Can you work these out from the model? Positions are in its coordinate system, mm. A direction names the side the tool comes from. Give positions to 0.01 mm unless a question says otherwise; leave off trailing zeros. Order: outer loops, then holes, each group sorted by start corner. A loop starts at its lowest first (then second) coordinate and runs counter-clockwise, first axis right, second up. Notation, with made-up numbers: M 75.5,81 L 119.5,81 A16 ccw 119.5,101 Z; hole C -9.5,-17 d2. An arc over 180 degrees is marked long. One line per question, with ' | ' between items. Start each with the question number.
1) If we section it at A-A, the plane y = 67.5: Please give me the cut outline in (x, z).
2) If we section it at D-D, the plane y = 79: Please give me the cut outline in (x, z), plus the area to 3 significant figures.
3) If we section it at C-C, the plane x = -25: State how many separate pieces and enclosed holes the cut face has, plus the area to 3 significant figures.
4) Thinking about a two-plate mould opening in Z: for faces 5 (the flat face through (-57.2, 19, 178)), 6 (the flat face through (-55.93, 24.31, 181.27)), which applies, +Z half, -Z half, draft (parallel to the pull), parting line (faces both ways), or undercut?
5) If we section it at B-B, the plane z = 65.5: Please give me the cut outline in (x, y).
6) For faces 1 (the flat face through (-55.932, 18.14, 98.395)), 2 (the flat face through (-1, 27, 169)), 3 (the flat face through (56.132, 24.308, 242.731)), 4 (the conical face through (-36.364, 61.607, -2.188)), which set-ups out of +Z, -Z, +X, -X, +Y, -Y let a thin tool reach every point of the face, with its end or its side?
7) I'm going to push flat-ended pins straight in: pin 1 Ø3 at (x, z) = (38.5, 98.5) entering from +Y; pin 2 Ø2.5 at (y, z) = (53.5, -2) entering from +X; pin 3 Ø1.5 at (y, z) = (4, 34.5) entering from -X; pin 4 Ø1 at (x, z) = (21.5, 222) entering from -Y. Where does each tip first touch, or does it pass through?
8) Please list where these lines run through material, in increasing order: line 1 along Z through (x, y) = (-37.5, 33); line 2 along Z through (x, y) = (12, 25); line 3 along Z through (x, y) = (52.5, 51). Write a range as [from, to].
```python
from build123d import *

# Parameters (mm, degrees)
SKETCH005_R             = 0.855
SKETCH005_R_2           = 0.85
SKETCH005_W             = 69.6
SKETCH005_H             = 13.447006
SKETCH005_H_2           = 27.45073
SKETCH005_H_3           = 18.514511
SKETCH005_H_4           = 22.526123
SKETCH005_H_5           = 22.717146
SKETCH005_H_6           = 29.263161
SKETCH005_H_7           = 8.474735
PAD004_DEPTH            = 3
SKETCH007_W             = 35
SKETCH007_H             = 5
PAD006_DEPTH            = 65
PAD006_DEPTH_BACK       = 3
HOLE001_D               = 3.4
HOLE001_DEPTH           = 25
HOLE001_CSINK_D         = 8
HOLE001_CSINK_ANGLE     = 90
PAD007_DEPTH            = 2.5
SKETCH010_W             = 55
SKETCH010_H             = 4
SKETCH010_W_2           = 50
PAD008_DEPTH            = 109.6
SKETCH011_R             = 2.75
POCKET_DEPTH            = 5
SKETCH012_R             = 2.75
POCKET001_DEPTH         = 5
SKETCH013_R             = 2.75
POCKET002_DEPTH         = 5
SKETCH014_R             = 5.1
PAD009_DEPTH            = 97.65
SKETCH015_R             = 1.7
POCKET003_DEPTH         = 14
BODY001_PLACEMENT_ANGLE = 180


with BuildPart() as part:
    # Sketch005 → Pad004 (new body)
    with BuildSketch(Plane.XZ):
        Polygon((-54.8, 256.6), (-54.8, 20), (-54.8, 0), (54.8, 0), (54.8, 20), (54.8, 256.6), (54.8, 259), (-54.8, 259), align=None)
        with Locations((-44.8, 30)):
            Circle(SKETCH005_R, mode=Mode.SUBTRACT)
        with Locations((44.8, 30)):
            Circle(SKETCH005_R, mode=Mode.SUBTRACT)
        with Locations((-44.8, 112)):
            Circle(SKETCH005_R, mode=Mode.SUBTRACT)
        with Locations((44.8, 112)):
            Circle(SKETCH005_R, mode=Mode.SUBTRACT)
        with Locations((-44.8, 157)):
            Circle(SKETCH005_R, mode=Mode.SUBTRACT)
        with Locations((44.8, 157)):
            Circle(SKETCH005_R, mode=Mode.SUBTRACT)
        with Locations((-44.8, 135)):
            Circle(SKETCH005_R, mode=Mode.SUBTRACT)
        with Locations((44.8, 135)):
            Circle(SKETCH005_R, mode=Mode.SUBTRACT)
        with Locations((-44.8, 230)):
            Circle(SKETCH005_R, mode=Mode.SUBTRACT)
        with Locations((44.8, 230)):
            Circle(SKETCH005_R, mode=Mode.SUBTRACT)
        with Locations((-44.8, 94)):
            Circle(SKETCH005_R, mode=Mode.SUBTRACT)
        with Locations((44.8, 94)):
            Circle(SKETCH005_R_2, mode=Mode.SUBTRACT)
        with Locations((0, 156.235863)):
            Rectangle(SKETCH005_W, SKETCH005_H, mode=Mode.SUBTRACT)
        with Locations((0, 120.786995)):
            Rectangle(SKETCH005_W, SKETCH005_H_2, mode=Mode.SUBTRACT)
        with Locations((0, 229.742745)):
            Rectangle(SKETCH005_W, SKETCH005_H_3, mode=Mode.SUBTRACT)
        with Locations((0, 194.222427)):
            Rectangle(SKETCH005_W, SKETCH005_H_4, mode=Mode.SUBTRACT)
        with Locations((0, 70.621734)):
            Rectangle(SKETCH005_W, SKETCH005_H_5, mode=Mode.SUBTRACT)
        with Locations((0, 29.63158)):
            Rectangle(SKETCH005_W, SKETCH005_H_6, mode=Mode.SUBTRACT)
        with Locations((0, 93.844347)):
            Rectangle(SKETCH005_W, SKETCH005_H_7, mode=Mode.SUBTRACT)
    extrude(amount=-PAD004_DEPTH)

    # Sketch007 → Pad006 (join, two sides)
    with BuildSketch(Plane.XZ) as pad006_sk:
        with Locations((-37.3, -2.5)):
            Rectangle(SKETCH007_W, SKETCH007_H)
        with Locations((37.3, -2.5)):
            Rectangle(SKETCH007_W, SKETCH007_H)
    extrude(amount=PAD006_DEPTH)
    extrude(pad006_sk.sketch, amount=-PAD006_DEPTH_BACK)

    # Hole001
    with Locations(Plane.XY):
        with Locations((-37.3, -55), (37.3, -55)):
            CounterSinkHole(HOLE001_D / 2, HOLE001_CSINK_D / 2, depth=HOLE001_DEPTH, counter_sink_angle=HOLE001_CSINK_ANGLE)

    # Sketch009 (on DatumPlane) → Pad007 (join)
    with BuildSketch(Plane.YZ.offset(54.8)):
        Polygon((-41, -5), (3, -5), (3, 28), align=None)
        Polygon((-23, 1), (-3, 16), (-3, 1), align=None, mode=Mode.SUBTRACT)
        Polygon((3, 198), (3, 165), (-41, 165), align=None)
        Polygon((-23, 171), (-3, 186), (-3, 171), align=None, mode=Mode.SUBTRACT)
        Polygon((3, 226), (3, 259), (-41, 259), align=None)
        Polygon((-23, 253), (-3, 238), (-3, 253), align=None, mode=Mode.SUBTRACT)
        Polygon((3, 118), (3, 85), (-41, 85), align=None)
        Polygon((-23, 91), (-3, 106), (-3, 91), align=None, mode=Mode.SUBTRACT)
    pad007 = extrude(amount=PAD007_DEPTH)

    # Mirrored001: Pad007 across YZ
    add(pad007.mirror(Plane.YZ))

    # Sketch010 (on DatumPlane) → Pad008 (join)
    with BuildSketch(Plane.YZ.offset(54.8)):
        with Locations((-27.5, 87)):
            Rectangle(SKETCH010_W, SKETCH010_H)
        with Locations((-27.5, 257)):
            Rectangle(SKETCH010_W, SKETCH010_H)
        with Locations((-27.5, 167)):
            Rectangle(SKETCH010_W, SKETCH010_H)
        with Locations((-25, 7)):
            Rectangle(SKETCH010_W_2, SKETCH010_H)
    extrude(amount=-PAD008_DEPTH)

    # Sketch011 (on DatumPlane) → Pocket (cut)
    with BuildSketch(Plane.XY.offset(169)):
        with Locations((0, -27.5)):
            Circle(SKETCH011_R)
    extrude(amount=-POCKET_DEPTH, mode=Mode.SUBTRACT)

    # Sketch012 (on DatumPlane) → Pocket001 (cut)
    with BuildSketch(Plane.XY.offset(89)):
        with Locations((0, -32)):
            Circle(SKETCH012_R)
    extrude(amount=-POCKET001_DEPTH, mode=Mode.SUBTRACT)

    # Sketch013 (on DatumPlane) → Pocket002 (cut)
    with BuildSketch(Plane.XY.offset(9)):
        with Locations((0, -25)):
            Circle(SKETCH013_R)
    extrude(amount=-POCKET002_DEPTH, mode=Mode.SUBTRACT)

    # Sketch014 → Pad009 (join)
    with BuildSketch(Plane.XZ):
        with Locations((-49.7, 249.9)):
            Circle(SKETCH014_R)
        with Locations((49.7, 249.9)):
            Circle(SKETCH014_R)
    extrude(amount=PAD009_DEPTH)

    # Sketch015 (on DatumPlane) → Pocket003 (cut)
    with BuildSketch(Plane.XZ.offset(97.65)):
        with Locations((-49.7, 249.9)):
            Circle(SKETCH015_R)
        with Locations((49.7, 249.9)):
            Circle(SKETCH015_R)
    extrude(amount=-POCKET003_DEPTH, mode=Mode.SUBTRACT)


with BuildPart() as part_1:
    # Body001 placement: moved
    add(part.part.moved(Location((0.1, 5, 0))).rotate(Axis((0.1, 5, 0), (0, 0, 1)), BODY001_PLACEMENT_ANGLE))


solid = part_1.part
```
Results found:
1) outline: M -54.7,-5 L -19.7,-5 L -19.7,0 L -54.7,0 Z; C -49.6,249.9 d10.2; M 19.9,-5 L 54.9,-5 L 54.9,0 L 19.9,0 Z; C 49.8,249.9 d10.2
2) outline: C -49.6,249.9 d10.2; C 49.8,249.9 d10.2 | area: 163 mm²
3) separate pieces: 8 | enclosed holes: 0 | area: 1,550 mm²
4) face 5: draft | face 6: undercut
5) outline: M -54.7,2 L -34.7,2 L -34.7,5 L -54.7,5 Z; M 34.9,2 L 54.9,2 L 54.9,5 L 34.9,5 Z
6) face 1: +X, -X | face 2: +Y | face 3: +X, +Y | face 4: none
7) pin 1: stops at y = 5 | pin 2: stops at x = 54.9 | pin 3: stops at x = -54.7 | pin 4: passes through
8) line 1: z = [-5, 0], [5, 9], [85, 89], [165, 169], [255, 259] | line 2: z = [5, 9], [85, 89], [165, 169], [255, 259] | line 3: z = [-5, 0], [5, 9], [85, 89], [165, 169], [245.57, 254.23], [255, 259]
